Verification items for the finished model (mm, model axes). Give positions to 0.01 mm unless a question says otherwise; leave off trailing zeros. Write each loop counter-clockwise with the first axis right and the second up, starting at its lowest first coordinate (ties: lowest second). Pieces come first, ordered by that corner, then holes. Notation, with made-up numbers: M -11.75,33.5 L 33.25,33.5 A33 cw 33.25,69.5 Z; hole C 87,9 d8. An arc over 180 degrees is marked long. Answer as a JSON object with one key per item and string values.
```python
from build123d import *

# Parameters (mm, degrees)
SKETCH1_R           = 1.725
SKETCH1_R_2         = 3
BOSS_EXTRUDE1_DEPTH = 2
FILLET1_R           = 4


with BuildPart() as part:
    # Sketch1 → Boss-Extrude1 (new body)
    with BuildSketch(Plane.XY):
        with BuildLine():
            ThreePointArc((16.775756842, 22.418161887), (0, 28), (-16.775756842, 22.418161887))
            ThreePointArc((-16.775756842, 22.418161887), (-22.627416998, 22.627416998), (-22.418161887, 16.775756842))
            ThreePointArc((-22.418161887, 16.775756842), (-28, 0), (-22.418161887, -16.775756842))
            ThreePointArc((-22.418161887, -16.775756842), (-22.627416998, -22.627416998), (-16.775756842, -22.418161887))
            ThreePointArc((-16.775756842, -22.418161887), (0, -28), (16.775756842, -22.418161887))
            ThreePointArc((16.775756842, -22.418161887), (22.627416998, -22.627416998), (22.418161887, -16.775756842))
            ThreePointArc((22.418161887, -16.775756842), (28, 0), (22.418161887, 16.775756842))
            ThreePointArc((22.418161887, 16.775756842), (22.627416998, 22.627416998), (16.775756842, 22.418161887))
        make_face()
        with Locations((19.798989873, 19.798989873)):
            Circle(SKETCH1_R, mode=Mode.SUBTRACT)
        with Locations((-19.798989873, 19.798989873)):
            Circle(SKETCH1_R, mode=Mode.SUBTRACT)
        with Locations((-19.798989873, -19.798989873)):
            Circle(SKETCH1_R, mode=Mode.SUBTRACT)
        with Locations((19.798989873, -19.798989873)):
            Circle(SKETCH1_R, mode=Mode.SUBTRACT)
        with Locations((0, 13)):
            Circle(SKETCH1_R_2, mode=Mode.SUBTRACT)
        with Locations((0, -13)):
            Circle(SKETCH1_R_2, mode=Mode.SUBTRACT)
    extrude(amount=BOSS_EXTRUDE1_DEPTH)

    # Fillet1
    fillet1_edges = [part.edges().sort_by_distance(p)[0] for p in [
        (-22.418161887, 16.775756842, 1),
        (-16.775756842, 22.418161887, 1),
        (16.775756842, 22.418161887, 1),
        (22.418161887, 16.775756842, 1),
        (22.418161887, -16.775756842, 1),
        (16.775756842, -22.418161887, 1),
        (-16.775756842, -22.418161887, 1),
        (-22.418161887, -16.775756842, 1),
    ]]
    fillet(fillet1_edges, radius=FILLET1_R)


solid = part.part
```
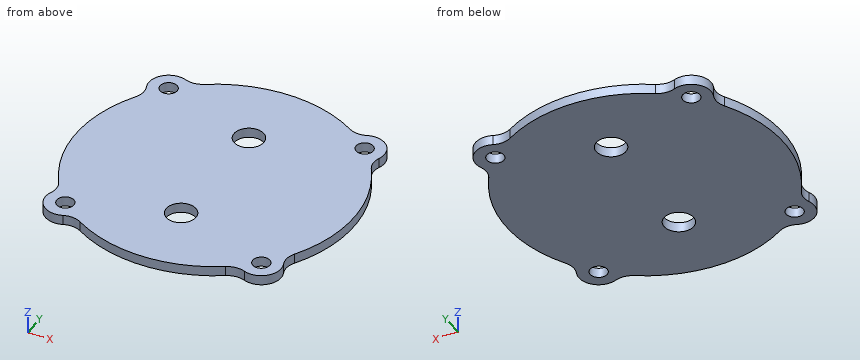
1) Section check A-A on x = 0. Record the boundary of the cut face in (y, z), and give its area (3 significant figures).
Completed:
{"outline": "M -28,0 L -16,0 L -16,2 L -28,2 Z; M -10,0 L 10,0 L 10,2 L -10,2 Z; M 16,0 L 28,0 L 28,2 L 16,2 Z", "area": "88.0 mm2"}
2) Thickness scan on L1, parallel to Y at x = 0, z = 1.6; L2, parallel to Y at x = 2, z = 0.3; L3, parallel to X at y = 12, z = 0.6. Record the ranges inside material, lowest first.
Completed:
{"L1": "y = -28 to -16, -10 to 10, 16 to 28", "L2": "y = -27.93 to -15.24, -10.76 to 10.76, 15.24 to 27.93", "L3": "x = -25.3 to -2.83, 2.83 to 25.3"}
3) Go/stop test with a flat-tipped pin: pin 1 (3 mm diameter, centred on x = 19.8, y = -19.8, fed in from -Z). Record where the tip stops, or that it passes through.
Completed:
{"pin 1": "passes through"}
4) Section check B-B on y = 13. Record the boundary of the cut face in (x, z), and give its area (3 significant figures).
Completed:
{"outline": "M -24.8,0 L -3,0 L -3,2 L -24.8,2 Z; M 3,0 L 24.8,0 L 24.8,2 L 3,2 Z", "area": "87.2 mm2"}
5) Section check C-C on z = 0.5. Count the separate pieces of the cut face and the enclosed holes in it, and give its area (3 significant figures).
Completed:
{"separate pieces": "1", "enclosed holes": "6", "area": "2,480 mm2"}
